Can you work these out from the drawing? Everything is in mm from the part's minimum corner. Coordinates: 2 decimals unless noted, no trailing zeros. Order: outer loops, then holes, each group sorted by start corner. A loop starts at its lowest first (then second) coordinate and runs counter-clockwise, first axis right, second up. Notation, with made-up numbers: M 77.5,43 L 90.5,43 A25 cw 90.5,73 Z; hole C -29.75,-7.75 d5. An arc over 180 degrees is marked long. Answer as CSV lines item,"result". Start each with the question number.
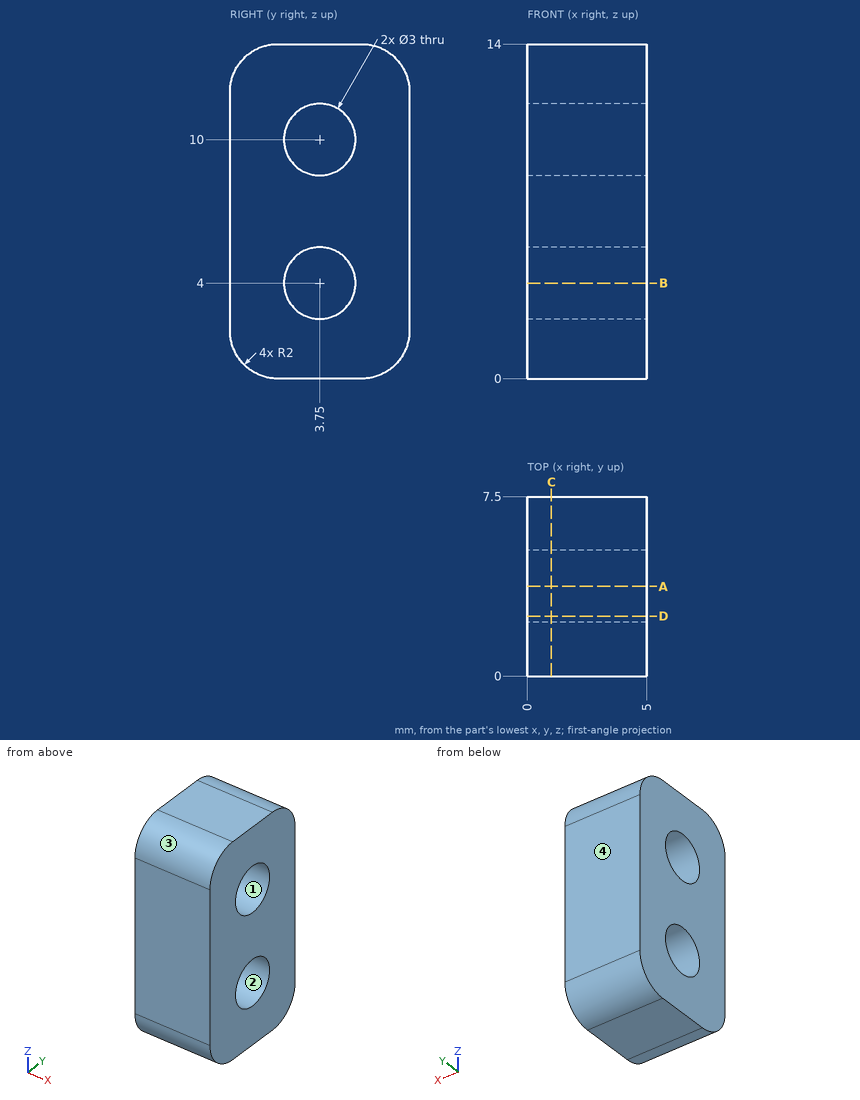
1) Suppose I cut it at D-D on y = 2.5. Please give me the cut outline in (x, z), plus the area to 3 significant figures.
2) Will this pin go through, and if not, where does the flat tip stop? pin 1 Ø1.8 at (y, z) = (3.75, 4) entering from -X.
3) Suppose I cut it at C-C on x = 1. Please give me the cut outline in (y, z).
4) Suppose I cut it at B-B on z = 4. Please give me the cut outline in (x, y), plus the area to 3 significant figures.
5) I need wall thicknesses on line 1 (Y direction, x = 1.15, z = 10); line 2 (Z direction, x = 0.4, y = 4); line 3 (Z direction, x = 0.85, y = 3). Which ranges of each line are inside material? Lowest first, please. Write a range as [from, to].
6) If we mould it in two halves opening along Z, with no side actions, what happens to the marked faces 1, 2, 3 and 4? For each: released by +Z, released by -Z, zero draft, split by the parting line, or undercut.
7) Suppose I cut it at A-A on y = 3.75. Please give me the cut outline in (x, z), plus the area to 3 significant figures.
Output:
1,outline,"M 0,0 L 5,0 L 5,3.17 L 0,3.17 Z; M 0,4.83 L 5,4.83 L 5,9.17 L 0,9.17 Z; M 0,10.83 L 5,10.83 L 5,14 L 0,14 Z"
1,area,"53.4 mm²"
2,pin 1,"through"
3,outline,"M 0,2 A2 ccw 2,0 L 5.5,0 A2 ccw 7.5,2 L 7.5,12 A2 ccw 5.5,14 L 2,14 A2 ccw 0,12 Z; hole C 3.75,4 d3; hole C 3.75,10 d3"
4,outline,"M 0,0 L 5,0 L 5,2.25 L 0,2.25 Z; M 0,5.25 L 5,5.25 L 5,7.5 L 0,7.5 Z"
4,area,"22.5 mm²"
5,line 1,"[0, 2.25], [5.25, 7.5]"
5,line 2,"[0, 2.52], [5.48, 8.52], [11.48, 14]"
5,line 3,"[0, 2.7], [5.3, 8.7], [11.3, 14]"
6,face 1,"undercut"
6,face 2,"undercut"
6,face 3,"released by +Z"
6,face 4,"zero draft"
7,outline,"M 0,0 L 5,0 L 5,2.5 L 0,2.5 Z; M 0,5.5 L 5,5.5 L 5,8.5 L 0,8.5 Z; M 0,11.5 L 5,11.5 L 5,14 L 0,14 Z"
7,area,"40.0 mm²"
